Job drawing, mm, ordinate dimensions from the low corner. One solid piece. Coordinates: 2 decimals unless noted, no trailing zeros. Write each loop counter-clockwise with the first axis right and the second up, starting at its lowest first coordinate (ties: lowest second). Pieces come first, ordered by that corner, then holes. Notation, with made-up numbers: (-26.5, 62.5) - (9.5, 62.5) arc R17 cw to (9.5, 79.5) - close; hole circle Ø10 at (38.5, 34). An arc over 180 degrees is marked (long way). Put each result on its own line as item: value. Start each with the question number.
1. Drop a flat-ended pin along its axis: P1, Ø1, axis at y = 5.5, z = 4, coming from the -X side. Give the stop position or say it passes through.
2. Saw through at A-A, the plane z = 3.55. Write the cut outline in (x, y).
3. Pull direction X, two halves, no side cores. Call the marked faces 1, 2, 3 and 4: released by +X, released by -X, zero draft, split by the parting line, or undercut.
4. Drill centre lines: L1, parallel to Y at x = 4, z = 2; L2, parallel to Y at x = 0.75, z = 1.65; L3, parallel to Y at x = 7, z = 2.65 (1 decimal). Where is each one in solid material? Low to high. Write a range as from..to.
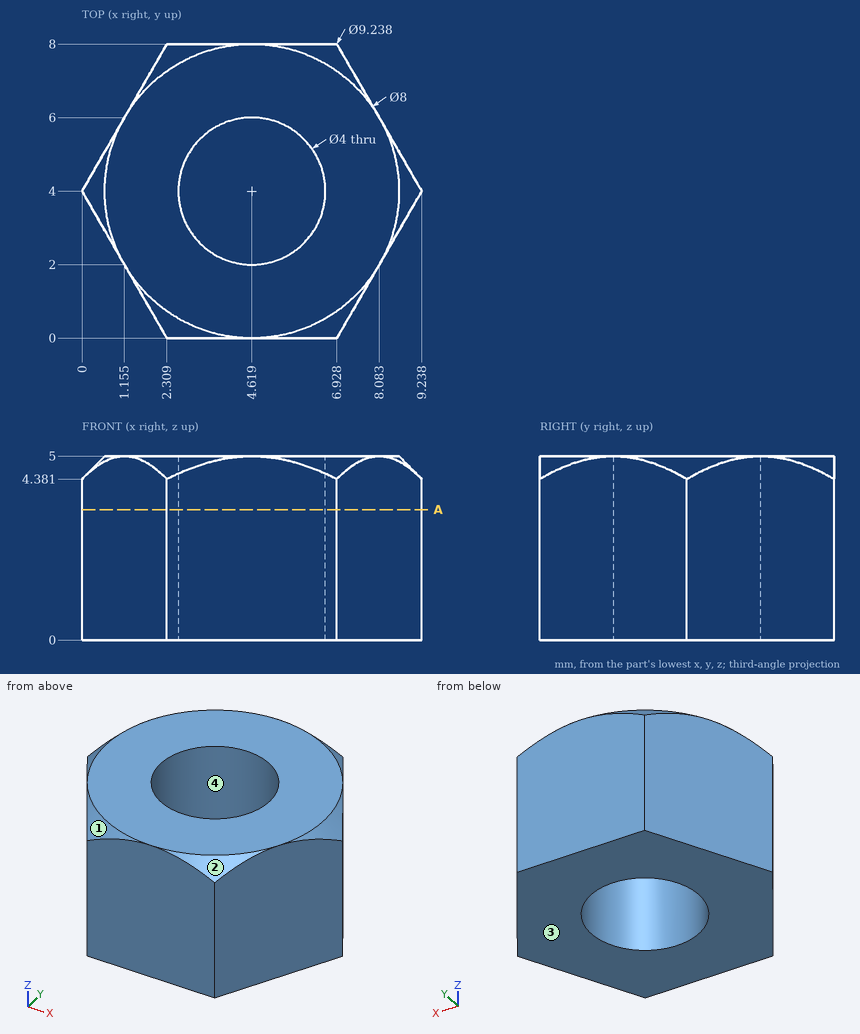
Final values:
1. P1: stops at x = 0.58
2. outline: (0, 4) - (2.31, 0) - (6.93, 0) - (9.24, 4) - (6.93, 8) - (2.31, 8) - close; hole circle Ø4 at (4.62, 4)
3. face 1: released by -X
3. face 2: released by +X
3. face 3: zero draft
3. face 4: undercut
4. L1: y = 0..2.1, 5.9..8
4. L2: y = 2.7..5.3
4. L3: y = 0.1..7.9
